The listing builds one solid part. Answer for the finished solid, in the listing's coordinates (mm). Round coordinates to 2 decimals unless told otherwise and drop trailing zeros. Loops run counter-clockwise (first coordinate to the right, second up) from the corner with the lowest first, then second, coordinate; pieces in that order, holes last. Notation, with made-up numbers: (79.5, 70.5) -> (105.5, 70.5) arc R20 ccw to (105.5, 79.5) -> close; hole circle Ø3 at (6.5, 1). An arc over 180 degrees is marked (long way). One line per question, with ' | ' between items.
Autodesk Inventor part; units mm, degrees
ref_plane "YZ Plane" through (0, 0, 0) normal (1, 0, 0) x (0, 1, 0)
ref_plane "XZ Plane" through (0, 0, 0) normal (0, 1, 0) x (-1, 0, 0)
ref_plane "XY Plane" through (0, 0, 0) normal (0, 0, 1) x (1, 0, 0)
sketch "Sketch4" plane through (0, 0, 0) normal (0, 1, 0) x (-1, 0, 0)
  circle A0 centre (0, 0) radius 6.35
  dimension "d10" = 12.7
extrude "Extrusion4" add sketch "Sketch4" along normal blind 745
sketch "Sketch5" plane through (0, 745, 0) normal (0, 1, 0) x (1, 0, 0)
  circle A0 centre (0, 0) radius 5.95
  circle A1 centre (0, 0) radius 6.35
  dimension "d13" = 11.9
extrude "Extrusion5" cut sketch "Sketch5" against normal blind 25
sketch "Sketch6" plane through (0, 0, 0) normal (0, -1, 0) x (1, 0, 0)
  circle A0 centre (0, 0) radius 6.35
  circle A1 centre (0, 0) radius 5.95
extrude "Extrusion6" cut sketch "Sketch6" against normal blind 40
properties part number "Eixotrifilado" material "Steel, Alloy"
Q1. Given pin 1 Ø5 at (y, z) = (481.5, -4.5) entering from +X; pin 2 Ø1 at (x, y) = (-3, 450.5) entering from +Z; pin 3 Ø6.5 at (x, z) = (3, -2) entering from -Y; pin 4 Ø1 at (x, y) = (5, 326.5) entering from -Z, each flat-ended and moving along its own axis, determine where each tip first touches the part or whether it passes through.
Numbers:
pin 1: x = 6.03 | pin 2: z = 5.84 | pin 3: y = 0 | pin 4: z = -4.48
Q2. Find the intervals of material crossed by line 1 (X direction, y = 620, z = -0.5); line 2 (Z direction, x = -2.5, y = 235); line 3 (Z direction, x = -1, y = 581), in increasing order. Write a range as from..to.
Numbers:
line 1: -6.33..6.33 | line 2: -5.84..5.84 | line 3: -6.27..6.27
Q3. A cutting plane is placed at B-B on z = 3.5. Give the vertices of the cut face in (x, y).
Numbers:
outline: (-5.3, 40) -> (-4.81, 40) -> (-4.81, 0) -> (4.81, 0) -> (4.81, 40) -> (5.3, 40) -> (5.3, 720) -> (4.81, 720) -> (4.81, 745) -> (-4.81, 745) -> (-4.81, 720) -> (-5.3, 720) -> close
Q4. A cutting plane is placed at A-A on x = 2.75. Give the vertices of the cut face in (y, z).
Numbers:
outline: (0, -5.28) -> (40, -5.28) -> (40, -5.72) -> (720, -5.72) -> (720, -5.28) -> (745, -5.28) -> (745, 5.28) -> (720, 5.28) -> (720, 5.72) -> (40, 5.72) -> (40, 5.28) -> (0, 5.28) -> close
Q5. A cutting plane is placed at C-C on y = 473. Give the vertices of the cut face in (x, z).
Numbers:
outline: circle Ø12.7 at (0, 0)
